from build123d import *

# Parameters (mm, degrees)
SKETCH1_W                      = 168
SKETCH1_H                      = 63
BOSS_EXTRUDE1_DEPTH            = 10
SKETCH2_W                      = 168
SKETCH2_H                      = 63
BOSS_EXTRUDE2_DEPTH            = 2
SKETCH3_W                      = 10
SKETCH3_H                      = 25
CUT_EXTRUDE1_DEPTH             = 111.028405423
SKETCH4_W                      = 10
SKETCH4_H                      = 8
CUT_EXTRUDE2_DEPTH             = 3
CUT_EXTRUDE2_DIRECTION_2_REACH = 114.236
SKETCH6_W                      = 10
SKETCH6_H                      = 1
BOSS_EXTRUDE4_DEPTH            = 31
SKETCH7_R                      = 1.5
BOSS_EXTRUDE5_DEPTH            = 3
SKETCH8_W                      = 10
SKETCH8_H                      = 5
BOSS_EXTRUDE6_DEPTH            = 3


with BuildPart() as part:
    # Sketch1 → Boss-Extrude1 (new body)
    with BuildSketch(Plane(origin=(0, 0, 0), x_dir=(1, 0, 0), z_dir=(0, 1, 0))):
        Polygon((0, 34.5), (-87, 34.5), (-87, -34.5), (84, -34.5), (104, -34.5), (104, 34.5), (84, 34.5), align=None)
        Rectangle(SKETCH1_W, SKETCH1_H, mode=Mode.SUBTRACT)
    extrude(amount=BOSS_EXTRUDE1_DEPTH)

    # Sketch2 → Boss-Extrude2 (add)
    with BuildSketch(Plane(origin=(0, 0, 0), x_dir=(1, 0, 0), z_dir=(0, 1, 0))):
        Rectangle(SKETCH2_W, SKETCH2_H)
    extrude(amount=BOSS_EXTRUDE2_DEPTH)

    # Sketch3 → Cut-Extrude1 (cut, through all)
    with BuildSketch(Plane(origin=(0, 10, 0), x_dir=(1, 0, 0), z_dir=(0, 1, 0))):
        with Locations((94, 19)):
            Rectangle(SKETCH3_W, SKETCH3_H)
    cut_extrude1 = extrude(amount=-CUT_EXTRUDE1_DEPTH, mode=Mode.SUBTRACT)

    # Mirror1: Cut-Extrude1 across plane
    add(cut_extrude1.mirror(Plane.XY), mode=Mode.SUBTRACT)

    # Sketch4 → Cut-Extrude2 (cut)
    with BuildSketch(Plane.XY.offset(6.5)):
        with Locations((94, 4)):
            Rectangle(SKETCH4_W, SKETCH4_H)
    cut_extrude2 = extrude(amount=-CUT_EXTRUDE2_DEPTH, mode=Mode.SUBTRACT)

    # Sketch4 → Cut-Extrude2 direction 2 (cut, up to next)
    with BuildSketch(Plane.XY.offset(6.5), mode=Mode.PRIVATE) as cut_extrude2_direction_2_sk1:
        with Locations((94, 4)):
            Rectangle(SKETCH4_W, SKETCH4_H)
    cut_extrude2_direction_2_tool1 = extrude(cut_extrude2_direction_2_sk1.sketch, amount=CUT_EXTRUDE2_DIRECTION_2_REACH, mode=Mode.PRIVATE) & part.part
    cut_extrude2_direction_2 = cut_extrude2_direction_2_tool1.solids().sort_by_distance((94, 4, 6.5))[0]
    add(cut_extrude2_direction_2, mode=Mode.SUBTRACT)

    # Mirror2: Cut-Extrude2, Cut-Extrude2 direction 2 across plane
    add(cut_extrude2.mirror(Plane.XY), mode=Mode.SUBTRACT)
    add(cut_extrude2_direction_2.mirror(Plane.XY), mode=Mode.SUBTRACT)

    # Sketch6 → Boss-Extrude4 (add)
    with BuildSketch(Plane.XY.offset(3.5)):
        with Locations((94, 0.5)):
            Rectangle(SKETCH6_W, SKETCH6_H)
    boss_extrude4 = extrude(amount=BOSS_EXTRUDE4_DEPTH)

    # Mirror5: Boss-Extrude4 across plane
    add(boss_extrude4.mirror(Plane.XY))

    # Sketch7 → Boss-Extrude5 (add)
    with BuildSketch(Plane.XY.offset(3.5)):
        with Locations((94, 4.5)):
            Circle(SKETCH7_R)
    boss_extrude5 = extrude(amount=BOSS_EXTRUDE5_DEPTH)

    # Mirror6: Boss-Extrude5 across plane
    add(boss_extrude5.mirror(Plane.XY))

    # Sketch8 → Boss-Extrude6 (add)
    with BuildSketch(Plane.ZY.offset(87)):
        with Locations((0, 2.5)):
            Rectangle(SKETCH8_W, SKETCH8_H)
    extrude(amount=BOSS_EXTRUDE6_DEPTH)


solid = part.part
Verification items for the finished model (mm, model axes). A direction names the side the tool comes from. Give positions to 0.01 mm unless a question says otherwise; leave off trailing zeros. Order: outer loops, then holes, each group sorted by start corner. A loop starts at its lowest first (then second) coordinate and runs counter-clockwise, first axis right, second up. Notation, with made-up numbers: M 16.25,15.25 L 29.25,15.25 A21 cw 29.25,30.25 Z; hole C 57,7.5 d5. An arc over 180 degrees is marked long. Answer as a JSON object with one key per item and string values. Group by question number.
1) Scan lines: line 1 along X through (y, z) = (6, 8.5); line 2 along X through (y, z) = (9, -4); line 3 along Z through (x, y) = (28, 3). Record each from-to range of solid material in increasing order. Write a range as [from, to].
2) Depth check by flat-ended pin: pin 1 Ø2.5 at (x, z) = (93, 32.5) entering from -Y; pin 2 Ø0.9 at (x, z) = (-88, 0) entering from +Y; pin 3 Ø2.5 at (x, y) = (93.5, 4) entering from +Z; pin 4 Ø2.5 at (y, z) = (4.5, -13) entering from -X. Enter the tip coordinate at first touch or a pass-through.
3) Cross-section at A-A (z = 0.5). Enter the section's corners in (x, y), then the cut area to 3 significant figures.
4) Mould release check, pull along Z, two halves, no side actions. Record for faces 1 (the face through (94, 1, -19)), 2 (the face through (7, 5, -34.5)), 3 (the face through (-1, 2, 0)): released by +Z, released by -Z, zero draft, split by the parting line, or undercut.
5) Cross-section at C-C (z = 8.5). Enter the section's corners in (x, y), then the cut area to 3 significant figures.
6) Access from +Z, -Z, +X, -X, +Y, -Y to the whole of each face (thin tool, end or side, straight path). Record for faces 4 (the face through (99, 5, -19)), 5 (the face through (94, 1, 19)), 6 (the face through (-1, 6, 31.5)), 7 (the face through (93, 3, -3.5)).
7) Cross-section at B-B (x = -44). Enter the section's corners in (y, z).
Result sheet:
{
 "1": {"line 1": "x = [-87, -84], [84, 89], [99, 104]", "line 2": "x = [-87, -84], [84, 104]", "line 3": "z = [-34.5, -31.5], [31.5, 34.5]"},
 "2": {"pin 1": "stops at y = 0", "pin 2": "stops at y = 5", "pin 3": "stops at z = 6.5", "pin 4": "stops at x = -87"},
 "3": {"outline": "M -90,0 L 104,0 L 104,10 L 84,10 L 84,2 L -84,2 L -84,10 L -87,10 L -87,5 L -90,5 Z", "area": "581 mm2"},
 "4": {"face 1": "zero draft", "face 2": "released by -Z", "face 3": "undercut"},
 "5": {"outline": "M -87,0 L 104,0 L 104,10 L 99,10 L 99,1 L 89,1 L 89,10 L 84,10 L 84,2 L -84,2 L -84,10 L -87,10 Z", "area": "476 mm2"},
 "6": {"face 4": "none", "face 5": "+Z", "face 6": "+Y", "face 7": "-Z"},
 "7": {"outline": "M 0,-34.5 L 10,-34.5 L 10,-31.5 L 2,-31.5 L 2,31.5 L 10,31.5 L 10,34.5 L 0,34.5 Z"}
}
